from build123d import *

# Parameters (mm, degrees)
F0_W     = 84
F0_H     = 102
F0_R     = 6
F1_DEPTH = 2
F2_R     = 5


with BuildPart() as f1:
    # F0 (on Top) → F1 (new body)
    with BuildSketch(Plane.XY):
        Rectangle(F0_W, F0_H)
        with BuildLine():
            Line((-25.050253, -41.414214), (-28.585786, -44.949747))
            ThreePointArc((-28.585786, -44.949747), (-34.949747, -44.949747), (-34.949747, -38.585786))
            Line((-34.949747, -38.585786), (-31.414214, -35.050253))
            ThreePointArc((-31.414214, -35.050253), (-25.050253, -35.050253), (-25.050253, -41.414214))
        make_face(mode=Mode.SUBTRACT)
        with BuildLine():
            ThreePointArc((25.050253, -41.414214), (25.050253, -35.050253), (31.414214, -35.050253))
            Line((31.414214, -35.050253), (34.949747, -38.585786))
            ThreePointArc((34.949747, -38.585786), (34.949747, -44.949747), (28.585786, -44.949747))
            Line((28.585786, -44.949747), (25.050253, -41.414214))
        make_face(mode=Mode.SUBTRACT)
        with BuildLine():
            ThreePointArc((-34.949747, 38.585786), (-34.949747, 44.949747), (-28.585786, 44.949747))
            Line((-28.585786, 44.949747), (-25.050253, 41.414214))
            ThreePointArc((-25.050253, 41.414214), (-25.050253, 35.050253), (-31.414214, 35.050253))
            Line((-31.414214, 35.050253), (-34.949747, 38.585786))
        make_face(mode=Mode.SUBTRACT)
        Circle(F0_R, mode=Mode.SUBTRACT)
        with BuildLine():
            Line((25.050253, 41.414214), (28.585786, 44.949747))
            ThreePointArc((28.585786, 44.949747), (34.949747, 44.949747), (34.949747, 38.585786))
            Line((34.949747, 38.585786), (31.414214, 35.050253))
            ThreePointArc((31.414214, 35.050253), (25.050253, 35.050253), (25.050253, 41.414214))
        make_face(mode=Mode.SUBTRACT)
    extrude(amount=F1_DEPTH)

    # F2
    f2_edges = [f1.edges().sort_by_distance(p)[0] for p in [
        (42, -51, 1),
        (42, 51, 1),
        (-42, -51, 1),
        (-42, 51, 1),
    ]]
    fillet(f2_edges, radius=F2_R)


solid = f1.part
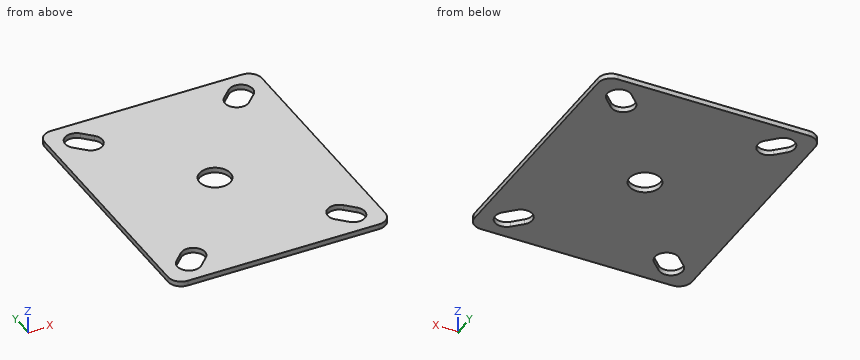
Design review of the part built by this model. Coordinates are the model's own, in mm. Give positions to 0.01 mm unless a question says otherwise; leave off trailing zeros. Loops run counter-clockwise (first coordinate to the right, second up) from the corner with the lowest first, then second, coordinate; pieces in that order, holes last. Notation, with made-up numbers: M 55,81.5 L 73,81.5 A14 ccw 73,88.5 Z; hole C -11.5,63.5 d11. An arc over 180 degrees is marked long. Answer as a JSON object with one key per item and string values.
Item 1: Wall thickness on line 1 along X through (y, z) = (-40, 0.8); line 2 along Y through (x, z) = (27, 1.55); line 3 along Y through (x, z) = (0, 1.5): over which ranges is each line inside the solid? List them lowest first.
Output values:
{"line 1": "x = -42 to -35.91, -24.09 to 24.09, 35.91 to 42", "line 2": "y = -51 to -43.36, -33.9 to 33.9, 43.36 to 51", "line 3": "y = -51 to -6, 6 to 51"}
Item 2: We need section C-C (z = 0.45). State the section outline as (x, y) points.
Output values:
{"outline": "M -42,-46 A5 ccw -37,-51 L 37,-51 A5 ccw 42,-46 L 42,46 A5 ccw 37,51 L -37,51 A5 ccw -42,46 Z; hole M -34.95,-38.59 A4.5 ccw -28.59,-44.95 L -25.05,-41.41 A4.5 ccw -31.41,-35.05 Z; hole M -34.95,38.59 L -31.41,35.05 A4.5 ccw -25.05,41.41 L -28.59,44.95 A4.5 ccw Z; hole C 0,0 d12; hole M 25.05,-41.41 L 28.59,-44.95 A4.5 ccw 34.95,-38.59 L 31.41,-35.05 A4.5 ccw Z; hole M 25.05,41.41 A4.5 ccw 31.41,35.05 L 34.95,38.59 A4.5 ccw 28.59,44.95 Z"}
Item 3: We need section B-B (y = 0). State the section outline as (x, z) points, and give its area (3 significant figures).
Output values:
{"outline": "M -42,0 L -6,0 L -6,2 L -42,2 Z; M 6,0 L 42,0 L 42,2 L 6,2 Z", "area": "144 mm2"}
Item 4: We need section A-A (x = 0). State the section outline as (y, z) points, and give its area (3 significant figures).
Output values:
{"outline": "M -51,0 L -6,0 L -6,2 L -51,2 Z; M 6,0 L 51,0 L 51,2 L 6,2 Z", "area": "180 mm2"}
